from build123d import *

# Parameters (mm, degrees)
BASE_DEPTH                      = 3
ESQUISSE3_W                     = 20.2
ESQUISSE3_H                     = 20.2
ENL_V_MAT_EXTRU_1_DEPTH         = 4
R_P_TITION_LIN_AIRE1_COUNT      = 2
R_P_TITION_LIN_AIRE1_PITCH      = 267.5
R_P_TITION_LIN_AIRE1_COUNT_DIR2 = 2
R_P_TITION_LIN_AIRE1_PITCH_DIR2 = 116
ESQUISSE4_R                     = 35
ENL_V_MAT_EXTRU_2_DEPTH         = 4
ESQUISSE5_R                     = 6
ESQUISSE5_W                     = 30
ESQUISSE5_H                     = 10
ENL_V_MAT_EXTRU_3_DEPTH         = 4
ESQUISSE6_R                     = 1.625
ENL_V_MAT_EXTRU_4_DEPTH         = 4
SKETCH1_W                       = 3
SKETCH1_H                       = 10
CUT_EXTRUDE1_DEPTH              = 4
LPATTERN1_COUNT                 = 4
LPATTERN1_PITCH                 = 20
SKETCH2_W                       = 3
SKETCH2_H                       = 10
CUT_EXTRUDE2_DEPTH              = 4
LPATTERN2_COUNT                 = 5
LPATTERN2_PITCH                 = 20
SKETCH4_W                       = 3
SKETCH4_H                       = 10
CUT_EXTRUDE3_DEPTH              = 4
LPATTERN3_COUNT                 = 2
LPATTERN3_PITCH                 = 20
ESQUISSE7_W                     = 10
ESQUISSE7_H                     = 3
ENL_V_MAT_EXTRU_5_DEPTH         = 3
ESQUISSE8_W                     = 3
ESQUISSE8_H                     = 10
ENL_V_MAT_EXTRU_6_DEPTH         = 3


with BuildPart() as part:
    # Esquisse1 → Base (new body)
    with BuildSketch(Plane.XY):
        Polygon((24.748737342, 24.748737342), (0, 0), (-150, 0), (-174.748737342, 24.748737342), (-174.748737342, 274.748737342), (-150, 299.497474683), (0, 299.497474683), (24.748737342, 274.748737342), align=None)
    extrude(amount=BASE_DEPTH)

    # Esquisse3 → Enlèv. mat.-Extru.1 (cut, through all)
    with BuildSketch(Plane.XY.offset(3)):
        with Locations((-132.998737342, 16)):
            Rectangle(ESQUISSE3_W, ESQUISSE3_H)
    enl_v_mat_extru_1 = extrude(amount=-ENL_V_MAT_EXTRU_1_DEPTH, mode=Mode.SUBTRACT)

    # Répétition linéaire1: Enl_v. mat.-Extru.1 2 × 2
    with Locations(*[(j * R_P_TITION_LIN_AIRE1_PITCH_DIR2, i * R_P_TITION_LIN_AIRE1_PITCH, 0) for i in range(R_P_TITION_LIN_AIRE1_COUNT) for j in range(R_P_TITION_LIN_AIRE1_COUNT_DIR2) if (i, j) != (0, 0)]):
        add(enl_v_mat_extru_1, mode=Mode.SUBTRACT)

    # Esquisse4 → Enlèv. mat.-Extru.2 (cut, through all)
    with BuildSketch(Plane.XY.offset(3)):
        with Locations((-15.251262658, 159.497474683)):
            Circle(ESQUISSE4_R)
    extrude(amount=-ENL_V_MAT_EXTRU_2_DEPTH, mode=Mode.SUBTRACT)

    # Esquisse5 → Enlèv. mat.-Extru.3 (cut, through all)
    with BuildSketch(Plane.XY.offset(3)):
        with Locations((-75, 30)):
            Circle(ESQUISSE5_R)
        with Locations((-75, 269.497474683)):
            Circle(ESQUISSE5_R)
        with Locations((-75, 149.748737342)):
            Rectangle(ESQUISSE5_W, ESQUISSE5_H)
    extrude(amount=-ENL_V_MAT_EXTRU_3_DEPTH, mode=Mode.SUBTRACT)

    # Esquisse6 → Enlèv. mat.-Extru.4 (cut, through all)
    with BuildSketch(Plane.XY.offset(3)):
        with Locations((-164.748737342, 249.497474683)):
            Circle(ESQUISSE6_R)
        with Locations((-141.748737342, 249.497474683)):
            Circle(ESQUISSE6_R)
        with Locations((-164.748737342, 50)):
            Circle(ESQUISSE6_R)
        with Locations((-141.748737342, 50)):
            Circle(ESQUISSE6_R)
    extrude(amount=-ENL_V_MAT_EXTRU_4_DEPTH, mode=Mode.SUBTRACT)

    # Sketch1 → Cut-Extrude1 (cut, through all)
    with BuildSketch(Plane.XY.offset(3)):
        with Locations((-16.998737342, 263.4)):
            Rectangle(SKETCH1_W, SKETCH1_H)
    cut_extrude1 = extrude(amount=-CUT_EXTRUDE1_DEPTH, mode=Mode.SUBTRACT)

    # LPattern1: Cut-Extrude1 ×4
    with Locations(*[(0, -i * LPATTERN1_PITCH, 0) for i in range(1, LPATTERN1_COUNT)]):
        add(cut_extrude1, mode=Mode.SUBTRACT)

    # Sketch2 → Cut-Extrude2 (cut, through all)
    with BuildSketch(Plane.XY.offset(3)):
        with Locations((-16.998737342, 36.1)):
            Rectangle(SKETCH2_W, SKETCH2_H)
    cut_extrude2 = extrude(amount=-CUT_EXTRUDE2_DEPTH, mode=Mode.SUBTRACT)

    # LPattern2: Cut-Extrude2 ×5
    with Locations(*[(0, i * LPATTERN2_PITCH, 0) for i in range(1, LPATTERN2_COUNT)]):
        add(cut_extrude2, mode=Mode.SUBTRACT)

    # Sketch4 → Cut-Extrude3 (cut, through all)
    with BuildSketch(Plane.XY.offset(3)):
        with Locations((-132.998737342, 36.1)):
            Rectangle(SKETCH4_W, SKETCH4_H)
    cut_extrude3 = extrude(amount=-CUT_EXTRUDE3_DEPTH, mode=Mode.SUBTRACT)

    # LPattern3: Cut-Extrude3 ×2
    with Locations(*[(0, i * LPATTERN3_PITCH, 0) for i in range(1, LPATTERN3_COUNT)]):
        add(cut_extrude3, mode=Mode.SUBTRACT)

    # Esquisse7 → Enlèv. mat.-Extru.5 (cut)
    with BuildSketch(Plane.XY.offset(3)):
        with Locations((4.498737342, 122.6)):
            Rectangle(ESQUISSE7_W, ESQUISSE7_H)
        with Locations((-15.501262658, 196.897474683)):
            Rectangle(ESQUISSE7_W, ESQUISSE7_H)
        with Locations((4.498737342, 196.897474683)):
            Rectangle(ESQUISSE7_W, ESQUISSE7_H)
        with Locations((-15.501262658, 122.6)):
            Rectangle(ESQUISSE7_W, ESQUISSE7_H)
    extrude(amount=-ENL_V_MAT_EXTRU_5_DEPTH, mode=Mode.SUBTRACT)

    # Esquisse8 → Enlèv. mat.-Extru.6 (cut)
    with BuildSketch(Plane.XY.offset(3)):
        with Locations((-52.001262658, 159.1)):
            Rectangle(ESQUISSE8_W, ESQUISSE8_H)
        with Locations((-52.001262658, 139.1)):
            Rectangle(ESQUISSE8_W, ESQUISSE8_H)
        with Locations((-52.001262658, 179.1)):
            Rectangle(ESQUISSE8_W, ESQUISSE8_H)
    extrude(amount=-ENL_V_MAT_EXTRU_6_DEPTH, mode=Mode.SUBTRACT)


solid = part.part
Design review of the part built by this model. Coordinates are the model's own, in mm. Give positions to 0.01 mm unless a question says otherwise; leave off trailing zeros. Loops run counter-clockwise (first coordinate to the right, second up) from the corner with the lowest first, then second, coordinate; pieces in that order, holes last. Notation, with made-up numbers: M -31.75,-32.5 L -22.75,-32.5 A13 cw -22.75,-10.5 Z; hole C 36,25 d6. An arc over 180 degrees is marked long. Write item = value, one per line.
Q1. We need section B-B (x = -75). Give the boundary of the cut face in (y, z), plus the area to 3 significant figures.
Output values:
outline = M 0,0 L 24,0 L 24,3 L 0,3 Z; M 36,0 L 144.75,0 L 144.75,3 L 36,3 Z; M 154.75,0 L 263.5,0 L 263.5,3 L 154.75,3 Z; M 275.5,0 L 299.5,0 L 299.5,3 L 275.5,3 Z
area = 796 mm^2
Q2. Draft analysis for pull direction Y (two halves, no side actions). For faces 1 (the cylindrical face through (-80.994, 269.761, 1.521)), 2 (the flat face through (-96, 152, 3)), 3 (the flat face through (13, 13, 1)), state which applies: +Y half, -Y half, draft (parallel to the pull), parting line (faces both ways), or undercut.
Output values:
face_1 = undercut
face_2 = draft
face_3 = -Y half
Q3. We need section A-A (y = 225). Give the boundary of the cut face in (x, z), plus the area to 3 significant figures.
Output values:
outline = M -174.75,0 L -18.5,0 L -18.5,3 L -174.75,3 Z; M -15.5,0 L 24.75,0 L 24.75,3 L -15.5,3 Z
area = 589 mm^2
Q4. Insertion check: pin 1 (0.9 mm diameter, centred on y = 19.5, z = 1.5, fed in from +X); pin 2 (1.5 mm diameter, centred on x = -16.5, z = 2, fed in from -Y); pin 3 (0.9 mm diameter, centred on x = 2.5, z = 2, fed in from -Y). Each pin has a flat end and moves straight along its axis. Give the tip position at first contact, or say it passes through.
Output values:
pin_1 = 19.95
pin_2 = 0
pin_3 = 2.05
Q5. We need section D-D (y = 139). Give the boundary of the cut face in (x, z).
Output values:
outline = M -174.75,0 L -53.5,0 L -53.5,3 L -174.75,3 Z; M -50.5,0 L -43.62,0 L -43.62,3 L -50.5,3 Z; M 13.12,0 L 24.75,0 L 24.75,3 L 13.12,3 Z
Q6. To check wall thickness, follow line 1 (Y direction, x = -75, z = 1.05); line 2 (Y direction, x = -137.5, z = 1.5); line 3 (Y direction, x = -65.5, z = 0.85). State the ranges of each line that lie inside material, in increasing order. Write a range as [from, to].
Output values:
line_1 = [0, 24], [36, 144.75], [154.75, 263.5], [275.5, 299.5]
line_2 = [0, 5.9], [26.1, 273.4], [293.6, 299.5]
line_3 = [0, 144.75], [154.75, 299.5]
Q7. We need section C-C (x = -4). Give the boundary of the cut face in (y, z), plus the area to 3 significant figures.
Output values:
outline = M 0,0 L 126.36,0 L 126.36,3 L 0,3 Z; M 192.64,0 L 299.5,0 L 299.5,3 L 192.64,3 Z
area = 700 mm^2
